```python
from build123d import *

# Parameters (mm, degrees)
BOSS_EXTRU_1_DEPTH           = 30
ESQUISSE3_R                  = 1
ENL_V_MAT_EXTRU_1_DEPTH      = 44.0464865
ESQUISSE4_R                  = 1.2
ENL_V_MAT_EXTRU_2_DEPTH      = 44.0464865
CONG_1_R                     = 2
ESQUISSE2_R                  = 1.2
BOSS_EXTRU_2_DEPTH           = 4
CONG_2_R                     = 1.5
ENL_V_MAT_EXTRU_3_DEPTH      = 44.04648657
ENL_V_MAT_EXTRU_3_DEPTH_BACK = 1
ESQUISSE5_R                  = 2.5
CHANFREIN1_SIZE              = 4
CHANFREIN1_SIZE_2            = 2.309401077


with BuildPart() as part:
    # Esquisse1 → Boss.-Extru.1 (new body)
    with BuildSketch(Plane.XY):
        with BuildLine():
            Line((0, 0), (-28, 0))
            Line((-28, 0), (-28, -4.803847577))
            Line((-28, -4.803847577), (-27.467711697, -5.725797963))
            ThreePointArc((-27.467711697, -5.725797963), (-21.449295844, -6.95), (-23.398313707, -12.774202037))
            Line((-23.398313707, -12.774202037), (-23.267949192, -13))
            Line((-23.267949192, -13), (-13.086942826, -13))
            Line((-13.086942826, -13), (-11.5, -4))
            Line((-11.5, -4), (0, -4))
            Line((0, -4), (0, 0))
        make_face()
    extrude(amount=BOSS_EXTRU_1_DEPTH)

    # Esquisse3 → Enlèv. mat.-Extru.1 (cut, through all)
    with BuildSketch(Plane(origin=(0, 0, 0), x_dir=(1, 0, 0), z_dir=(0, 1, 0))):
        with Locations(Location((-7.5, -8.5, 0), (0, 0, 180))):
            Circle(ESQUISSE3_R)
        with Locations(Location((-7.5, -21.5, 0), (0, 0, 180))):
            Circle(ESQUISSE3_R)
    extrude(amount=-ENL_V_MAT_EXTRU_1_DEPTH, mode=Mode.SUBTRACT)

    # Esquisse4 → Enlèv. mat.-Extru.2 (cut, through all)
    with BuildSketch(Plane.ZY):
        with Locations(Location((4.5, -9, 0), (0, 0, 180))):
            Circle(ESQUISSE4_R)
        with Locations(Location((25.5, -9, 0), (0, 0, 180))):
            Circle(ESQUISSE4_R)
    extrude(amount=ENL_V_MAT_EXTRU_2_DEPTH, mode=Mode.SUBTRACT)

    # Congé1
    cong_1_edges = [part.edges().sort_by_distance(p)[0] for p in [
        (-11.5, -4, 15),
        (-13.086942826, -13, 15),
        (-28, 0, 15),
    ]]
    fillet(cong_1_edges, radius=CONG_1_R)

    # Symétrie1: part across plane


with BuildPart() as part_1:
    add(part.part)
    add(part.part.mirror(Plane(origin=(0, -4, 30), x_dir=(0, 0, 1), z_dir=(-1, 0, 0))))

    # Esquisse2 → Boss.-Extru.2 (add)
    with BuildSketch(Plane(origin=(0, 0, 0), x_dir=(0, 0, -1), z_dir=(1, 0, 0))):
        with BuildLine():
            Line((0, 0), (-15.656854249, 0))
            Line((-15.656854249, 0), (-6.828427125, 8.828427125))
            ThreePointArc((-6.828427125, 8.828427125), (-2.469266271, 9.69551813), (0, 6))
            Line((0, 6), (0, 0))
        make_face()
        with Locations((-4, 6)):
            Circle(ESQUISSE2_R, mode=Mode.SUBTRACT)
    extrude(amount=BOSS_EXTRU_2_DEPTH)

    # Congé2
    cong_2_edges = [part_1.edges().sort_by_distance(p)[0] for p in [
        (4, 0, 7.828427125),
        (0, 0, 7.828427125),
        (2, 0, 15.656854249),
    ]]
    fillet(cong_2_edges, radius=CONG_2_R)

    # Esquisse5 → Enlèv. mat.-Extru.3 (cut, two sides: drawn at the far end of the back side and taken through both)
    with BuildSketch(Plane(origin=(0, 0, 0), x_dir=(1, 0, 0), z_dir=(0, 1, 0)).offset(-ENL_V_MAT_EXTRU_3_DEPTH_BACK)):
        with Locations((-7.5, -8.5)):
            Circle(ESQUISSE5_R)
        with Locations((-7.5, -21.5)):
            Circle(ESQUISSE5_R)
        with Locations(Location((7.5, -8.5, 0), (0, 0, 216.869897646))):
            Circle(ESQUISSE5_R)
        with Locations((7.5, -21.5)):
            Circle(ESQUISSE5_R)
    extrude(amount=ENL_V_MAT_EXTRU_3_DEPTH + ENL_V_MAT_EXTRU_3_DEPTH_BACK, mode=Mode.SUBTRACT)

    # Chanfrein1
    # the kernel refuses this chamfer: 4, 2.309401077 mm, written as the material it takes off along each edge
    with BuildSketch(Plane(origin=(-36.348343019, 0, 30), x_dir=(0, 0.019326765612700744, -0.9998132206222079), z_dir=(1, 0, 0))) as chanfrein1_piece_1:
        Polygon((CHANFREIN1_SIZE * 0.999813220622, -CHANFREIN1_SIZE * 0.0193267656127), (-CHANFREIN1_SIZE_2 * 0.0193267656107, -CHANFREIN1_SIZE_2 * 0.999813220518), (0, 0), align=None)
    extrude(amount=72.696686037, mode=Mode.SUBTRACT)


solid = part_1.part
```
For this review, take the finished solid that the model builds, in its own axes (mm). A direction names the side the tool comes from. Round coordinates to 2 decimals unless told otherwise and drop trailing zeros. Write each loop counter-clockwise with the first axis right and the second up, starting at its lowest first coordinate (ties: lowest second). Pieces come first, ordered by that corner, then holes. Notation, with made-up numbers: (-13, -7) - (12, -7) arc R14 cw to (12, 15) - close; hole circle Ø2 at (-23.75, -19.75). An arc over 180 degrees is marked (long way). Answer as a JSON object with one key per item and string values.
1. For pin 1 Ø5 at (x, y) = (-15.5, 4) entering from -Z; pin 2 Ø4 at (x, z) = (7.5, 8.5) entering from +Y; pin 3 Ø9.5 at (y, z) = (4, 8) entering from +X; pin 4 Ø6 at (x, z) = (1.5, 12.5) entering from -Y, all flat-tipped, find the tip position at first contact; note any pin that passes through.
Response values:
{"pin 1": "passes through", "pin 2": "stops at y = -1", "pin 3": "stops at x = 27.56", "pin 4": "stops at y = -4"}
2. We need section A-A on x = 7.5. Give the boundary of the cut face in (y, z).
Response values:
{"outline": "(-4, 0) - (0, 0) - (0, 6) - (-1, 6) - (-1, 7.5) - (-4, 7.5) - close; (-4, 9.5) - (-1, 9.5) - (-1, 11) - (0, 11) - (0, 19) - (-1, 19) - (-1, 20.5) - (-4, 20.5) - close; (-4, 22.5) - (-1, 22.5) - (-1, 24) - (0, 24) - (0, 26) - (-2.31, 30) - (-4, 30) - close"}
3. Tool access review of faces 1 (the face through (0, 5, 5)), 2 (the face through (5.08, -0.46, 9.12)), 3 (the face through (-0.392, -1.139, 27.972)), 4 (the face through (-12.3, -8.54, 14.79)): name each direction out of +Z, -Z, +X, -X, +Y, -Y from which nothing blocks a thin tool from reaching the whole face with its end or side.
Response values:
{"face 1": "+Z, -Z, -X, +Y", "face 2": "+Y", "face 3": "+Z, +X, -X, +Y", "face 4": "+Z, -Z, -Y"}
4. We need section B-B on x = 22.5. Give the boundary of the cut face in (y, z), then the cut area to 3 significant figures.
Response values:
{"outline": "(-13, 0) - (-12.25, 0) - (-12.25, 30) - (-13, 30) - close; (-5.75, 0) - (0, 0) - (0, 26) - (-2.31, 30) - (-5.75, 30) - close", "area": "190 mm2"}
5. Draft analysis for pull direction Z (two halves, no side actions). For faces 5 (the face through (-7.37, -2.48, 9.49)), 6 (the face through (0, -4, 15)), 7 (the face through (0, -3, 30)), state which applies: +Z half, -Z half, draft (parallel to the pull), parting line (faces both ways), or undercut.
Response values:
{"face 5": "undercut", "face 6": "draft", "face 7": "+Z half"}
6. We need section C-C on y = -9. Give the boundary of the cut face in (x, z).
Response values:
{"outline": "(-20.9, 0) - (-12.38, 0) - (-12.38, 3.3) - (-20.9, 3.3) - close; (-20.9, 5.7) - (-12.38, 5.7) - (-12.38, 24.3) - (-20.9, 24.3) - close; (-20.9, 26.7) - (-12.38, 26.7) - (-12.38, 30) - (-20.9, 30) - close; (12.38, 0) - (20.9, 0) - (20.9, 3.3) - (12.38, 3.3) - close; (12.38, 5.7) - (20.9, 5.7) - (20.9, 24.3) - (12.38, 24.3) - close; (12.38, 26.7) - (20.9, 26.7) - (20.9, 30) - (12.38, 30) - close"}
7. We need section D-D on x = 13.5. Give the boundary of the cut face in (y, z).
Response values:
{"outline": "(-12.55, 0) - (0, 0) - (0, 26) - (-2.31, 30) - (-12.55, 30) - close; hole circle Ø2.4 at (-9, 4.5); hole circle Ø2.4 at (-9, 25.5)"}
8. To check wall thickness, follow line 1 along Z through (x, y) = (15, -9); line 2 along Z through (x, y) = (19, -9.75); line 3 along Y through (x, z) = (-7.5, 2). State the ranges of each line that lie inside material, in increasing order.
Response values:
{"line 1": "z = 0 to 3.3, 5.7 to 24.3, 26.7 to 30", "line 2": "z = 0 to 3.56, 5.44 to 24.56, 26.44 to 30", "line 3": "y = -4 to 0"}
